from build123d import *

# Parameters (mm, degrees)
BOSS_EXTRUDE1_DEPTH = 3.175
CUT_EXTRUDE1_DEPTH  = 3.175
SKETCH3_W           = 3.175
SKETCH3_H           = 3.175
CUT_EXTRUDE2_DEPTH  = 3.175


with BuildPart() as part:
    # Sketch1 → Boss-Extrude1 (new body)
    with BuildSketch(Plane.XY):
        with BuildLine():
            Line((133.353452848, 0), (218.438559169, 0))
            Line((218.438559169, 0), (218.438559169, -3.175))
            Line((218.438559169, -3.175), (228.593504491, -3.175))
            Line((228.593504491, -3.175), (228.593504491, -41.275))
            Line((228.593504491, -41.275), (218.438559169, -41.275))
            Line((218.438559169, -41.275), (218.438559169, -44.45))
            Line((218.438559169, -44.45), (133.353452848, -44.45))
            add(Edge.make_bspline(
                [(133.353452848, 0), (129.670007688, -3.804094497), (126.127807653, -11.460398689), (125.717598982, -27.472957947), (126.742796491, -38.641939676), (133.353452848, -44.45)],
                knots=[0, 0, 0, 0, 0.328355513, 0.50111915, 1, 1, 1, 1], degree=3))
        make_face()
    extrude(amount=BOSS_EXTRUDE1_DEPTH)

    # Sketch2 → Cut-Extrude1 (cut)
    with BuildSketch(Plane.XY.offset(3.175)):
        with BuildLine():
            Line((135.939264538, 0), (128.336629453, 5.186344239))
            Line((128.336629453, 5.186344239), (108.478299615, -42.096060539))
            Line((108.478299615, -42.096060539), (132.091652271, -56.370762285))
            Line((132.091652271, -56.370762285), (135.939264538, -44.45))
            add(Edge.make_bspline(
                [(135.939264538, 0), (131.854984435, -6.817127359), (129.691129791, -22.368396799), (132.428444631, -37.615693349), (135.939264538, -44.45)],
                knots=[0, 0, 0, 0, 0.506942817, 1, 1, 1, 1], degree=3))
        make_face()
    extrude(amount=-CUT_EXTRUDE1_DEPTH, mode=Mode.SUBTRACT)

    # Sketch3 → Cut-Extrude2 (cut)
    with BuildSketch(Plane.XY.offset(3.175)):
        with Locations((140.231064965, -8.443013353)):
            Rectangle(SKETCH3_W, SKETCH3_H)
        with Locations((155.86048705, -5.370418658)):
            Rectangle(SKETCH3_W, SKETCH3_H)
        with Locations((147.789651456, -5.451485607)):
            Rectangle(SKETCH3_W, SKETCH3_H)
        with Locations((167.178168731, -5.087390187)):
            Rectangle(SKETCH3_W, SKETCH3_H)
        with Locations((179.891954361, -5.087390187)):
            Rectangle(SKETCH3_W, SKETCH3_H)
        with Locations((189.613004004, -5.451485607)):
            Rectangle(SKETCH3_W, SKETCH3_H)
        with Locations((199.872722139, -5.995153624)):
            Rectangle(SKETCH3_W, SKETCH3_H)
        with Locations((209.401626696, -38.454846376)):
            Rectangle(SKETCH3_W, SKETCH3_H)
        with Locations((199.872722139, -38.454846376)):
            Rectangle(SKETCH3_W, SKETCH3_H)
        with Locations((189.613004004, -38.998514393)):
            Rectangle(SKETCH3_W, SKETCH3_H)
        with Locations((179.891954361, -39.362609813)):
            Rectangle(SKETCH3_W, SKETCH3_H)
        with Locations((167.178168731, -39.362609813)):
            Rectangle(SKETCH3_W, SKETCH3_H)
        with Locations((147.789651456, -38.998514393)):
            Rectangle(SKETCH3_W, SKETCH3_H)
        with Locations((155.86048705, -39.079581342)):
            Rectangle(SKETCH3_W, SKETCH3_H)
        with Locations((140.231064965, -36.006986647)):
            Rectangle(SKETCH3_W, SKETCH3_H)
        with Locations((137.703428064, -29.629038879)):
            Rectangle(SKETCH3_W, SKETCH3_H)
        with Locations((137.703428064, -14.820961121)):
            Rectangle(SKETCH3_W, SKETCH3_H)
        with Locations((209.401626696, -5.995153624)):
            Rectangle(SKETCH3_W, SKETCH3_H)
    extrude(amount=-CUT_EXTRUDE2_DEPTH, mode=Mode.SUBTRACT)


solid = part.part
Can you work these out from the model? Positions are in its coordinate system, mm. Give positions to 0.01 mm unless a question says otherwise; leave off trailing zeros. Write each loop counter-clockwise with the first axis right and the second up, starting at its lowest first coordinate (ties: lowest second). Pieces come first, ordered by that corner, then holes. Notation, with made-up numbers: (10, -12.5) -> (16, -12.5) arc R22 ccw to (16, 4.5) -> close; hole circle Ø2 at (75, 85.25). An arc over 180 degrees is marked (long way). Answer as a JSON object with one key per item and string values. Group by question number.
Item 1: We'd pull the mould along X, two halves only. Please class faces 1 (the face through (228.594, -22, 2)), 2 (the face through (141.819, -8, 2)): +X half, -X half, draft (parallel to the pull), parting line (faces both ways), or undercut.
Item 2: Please list where these lines run through material, in increasing order: line 1 (Y direction, x = 139, z = 2.15); line 2 (Y direction, x = 190, z = 1.95); line 3 (Y direction, x = 179, z = 1.2). Write a range as [from, to].
Item 3: I'm going to push flat-ended pins straight in: P1, Ø1.6, axis at y = -39.5, z = 1, coming from the -X side; P2, Ø1, axis at x = 139.5, z = 1, coming from the +Y side. Where does each tip first touch, or does it pass through?
Item 4: Suppose I cut it at A-A (x = 156). Please give me the cut outline in (y, z) (3 decimals).
Item 5: Suppose I cut it at B-B (z = 0.7). State how many separate pieces and enclosed holes the cut face has, plus the area to 3 significant figures.
Item 6: Suppose I cut it at C-C (x = 221.5). Please give me the cut outline in (y, z) (3 decimals), plus the area to 3 significant figures.
Findings:
{
 "1": {"face 1": "+X half", "face 2": "undercut"},
 "2": {"line 1": "y = [-44.45, -37.59], [-34.42, -31.22], [-28.04, -16.41], [-13.23, -10.03], [-6.86, 0]", "line 2": "y = [-44.45, -40.59], [-37.41, -7.04], [-3.86, 0]", "line 3": "y = [-44.45, -40.95], [-37.78, -6.67], [-3.5, 0]"},
 "3": {"P1": "stops at x = 133.52", "P2": "stops at y = 0"},
 "4": {"outline": "(-44.45, 0) -> (-40.667, 0) -> (-40.667, 3.175) -> (-44.45, 3.175) -> close; (-37.492, 0) -> (-6.958, 0) -> (-6.958, 3.175) -> (-37.492, 3.175) -> close; (-3.783, 0) -> (0, 0) -> (0, 3.175) -> (-3.783, 3.175) -> close"},
 "5": {"separate pieces": "1", "enclosed holes": "18", "area": "4,030 mm²"},
 "6": {"outline": "(-41.275, 0) -> (-3.175, 0) -> (-3.175, 3.175) -> (-41.275, 3.175) -> close", "area": "121 mm²"}
}
